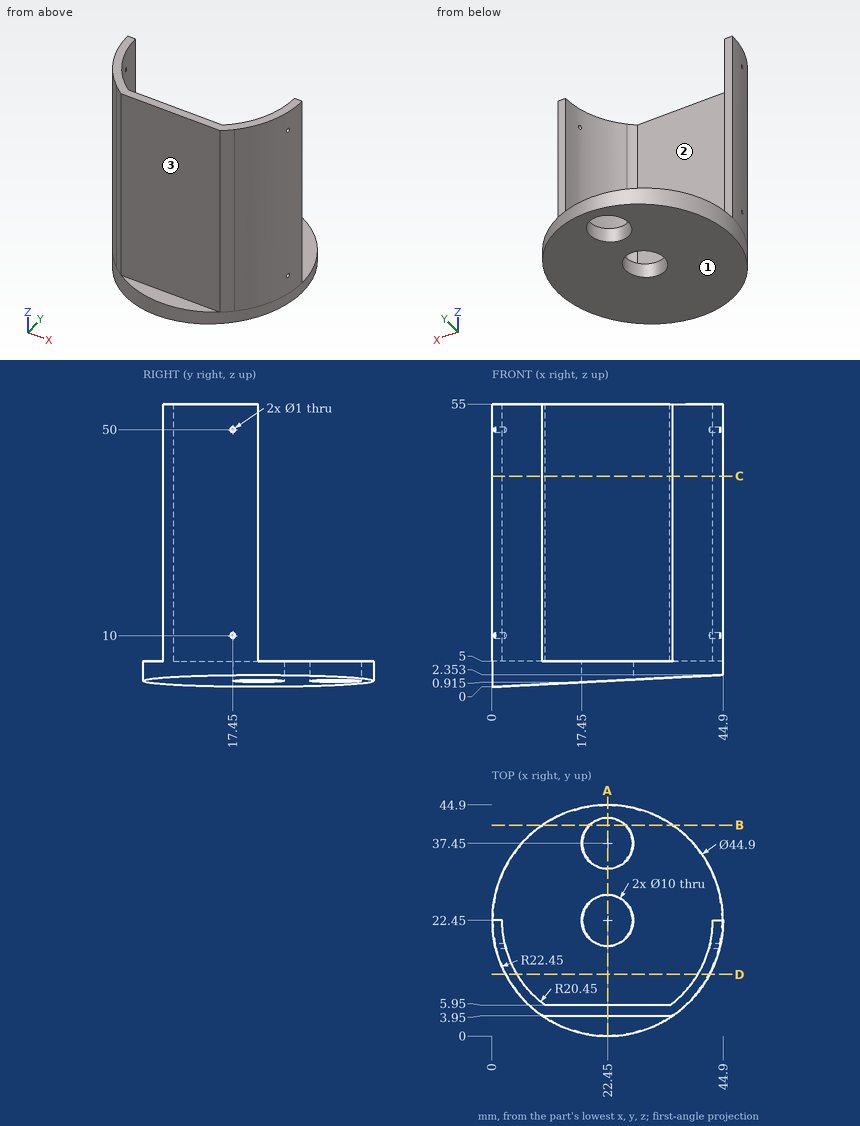
Drawing for the job (mm, zero at the part's lowest x, y, z). A direction names the side the tool comes from. Coordinates: 2 decimals unless noted, no trailing zeros. Order: outer loops, then holes, each group sorted by start corner. A loop starts at its lowest first (then second) coordinate and runs counter-clockwise, first axis right, second up. Notation, with made-up numbers: (66, 38) - (79, 38) arc R22 cw to (79, 49) - close; hole circle Ø1 at (-0.5, 86). An arc over 180 degrees is marked (long way). Use a Markdown table: item, result. Add a question column.
(1) Saw through at A-A (x = 22.45). Give the cut face in (y, z), then the cut area to 3 significant figures.
(2) Saw through at C-C (z = 41). Give the cut face in (x, y).
(3) Saw through at D-D (y = 12). Give the cut face in (x, z) (1 decimal).
(4) Drill centre lines: line 1 along Y through (x, z) = (22.45, 2.35); line 2 along Y through (x, z) = (20.5, 22.5); line 3 along Z through (x, y) = (43.3, 17.45). Where is each one in solid material? Low to high. Write a range as [from, to].
(5) Which spindle directions (+Z, -Z, +X, -X, +Y, -Y) get a long thin tool onto all of the face, cutting with end or side? Do the marked faces 1, 2 and 3. Say none if no direction does.
(6) Saw through at B-B (y = 41). Give the cut face in (x, z) (1 decimal).
(7) Flat gauge pins, fed straight in: pin 1 (1.5 mm diameter, centred on x = 37, z = 31.5, fed in from -Y); pin 2 (4 mm diameter, centred on x = 16.5, y = 20, fed in from -Z); pin 3 (12 mm diameter, centred on x = 12, z = 43.5, fed in from +Y); pin 4 (9 mm diameter, centred on x = 22.45, y = 22.45, fed in from -Z). Where does each tip first touch, or does it go through?
Solved:
| question | item | result |
|---|---|---|
| 1 | outline | (0, 1.18) - (17.45, 1.18) - (17.45, 5) - (5.95, 5) - (5.95, 55) - (3.95, 55) - (3.95, 5) - (0, 5) - close; (27.45, 1.18) - (32.45, 1.18) - (32.45, 5) - (27.45, 5) - close; (42.45, 1.18) - (44.9, 1.18) - (44.9, 5) - (42.45, 5) - close |
| 1 | area | 195 mm² |
| 2 | outline | (0, 22.45) arc R22.45 ccw to (9.73, 3.95) - (35.17, 3.95) arc R22.45 ccw to (44.9, 22.45) - (42.9, 22.45) arc R20.45 cw to (34.53, 5.95) - (10.37, 5.95) arc R20.45 cw to (2, 22.45) - close |
| 3 | outline | (2.6, 0.1) - (42.3, 2.2) - (42.3, 55) - (40, 55) - (40, 5) - (4.9, 5) - (4.9, 55) - (2.6, 55) - close |
| 4 | line 1 | y = [0, 17.45], [27.45, 32.45], [42.45, 44.9] |
| 4 | line 2 | y = [3.95, 5.95] |
| 4 | line 3 | z = [2.27, 9.5], [10.5, 49.5], [50.5, 55] |
| 5 | face 1 | -Z, +X, +Y, -Y |
| 5 | face 2 | +Z, +Y |
| 5 | face 3 | +Z, +X, -X, -Y |
| 6 | outline | (9.8, 0.5) - (18.9, 1) - (18.9, 5) - (9.8, 5) - close; (26, 1.4) - (35.1, 1.8) - (35.1, 5) - (26, 5) - close |
| 7 | pin 1 | stops at y = 4.74 |
| 7 | pin 2 | stops at z = 0.76 |
| 7 | pin 3 | stops at y = 10.3 |
| 7 | pin 4 | passes through |
